```python
from build123d import *

# Parameters (mm, degrees)
BOSS_EXTRUDE1_DEPTH = 3
CUT_EXTRUDE1_REACH  = 27.671
SKETCH4_R           = 2.5


with BuildPart() as part:
    # Sketch2 → Boss-Extrude1 (new body)
    with BuildSketch(Plane.XY):
        with BuildLine():
            Line((-20, 5), (20, 5))
            ThreePointArc((20, 5), (25, 0), (20, -5))
            Line((20, -5), (-20, -5))
            ThreePointArc((-20, -5), (-25, 0), (-20, 5))
        make_face()
    extrude(amount=BOSS_EXTRUDE1_DEPTH)

    # Sketch4 → Cut-Extrude1 (cut, up to next)
    with BuildSketch(Plane.XY.offset(3), mode=Mode.PRIVATE) as cut_extrude1_sk1:
        with Locations((-20, 0)):
            Circle(SKETCH4_R)
    cut_extrude1_tool1 = extrude(cut_extrude1_sk1.sketch, amount=-CUT_EXTRUDE1_REACH, mode=Mode.PRIVATE) & part.part
    # Sketch4 → Cut-Extrude1 (cut, up to next)
    with BuildSketch(Plane.XY.offset(3), mode=Mode.PRIVATE) as cut_extrude1_sk2:
        with BuildLine():
            Line((11, 2.5), (18, 2.5))
            ThreePointArc((18, 2.5), (20.5, 0), (18, -2.5))
            Line((18, -2.5), (11, -2.5))
            ThreePointArc((11, -2.5), (8.5, 0), (11, 2.5))
        make_face()
    cut_extrude1_tool2 = extrude(cut_extrude1_sk2.sketch, amount=-CUT_EXTRUDE1_REACH, mode=Mode.PRIVATE) & part.part
    add(cut_extrude1_tool1.solids().sort_by_distance((-20, 0, 3))[0], mode=Mode.SUBTRACT)
    add(cut_extrude1_tool2.solids().sort_by_distance((14.5, 0, 3))[0], mode=Mode.SUBTRACT)


solid = part.part
```
Source: CAD feature listing. Evaluate the final solid. Frame: model axes, mm. A direction names the side the tool comes from. Round coordinates to 2 decimals unless told otherwise and drop trailing zeros. Loops run counter-clockwise (first coordinate to the right, second up) from the corner with the lowest first, then second, coordinate; pieces in that order, holes last.
1. Contact query for a flat-ended pin moving along its axis: pin 1 (6 mm diameter, centred on x = 9, y = -1, fed in from +Z). Output: stop coordinate, or through.
2. Section query B-B on y = 0. Output: boundary loops of the cut face in (x, z), and give its area (3 significant figures).
3. Section query A-A on z = 1.2. Output: boundary loops of the cut face in (x, y), and give its area (3 significant figures).
4. Access query for faces 4 (the flat face through (0, 5, 1)), 5 (the flat face through (15, -2.5, 2)). Directions: +Z, -Z, +X, -X, +Y, -Y. A direction counts if a zero-diameter tool reaches every point of the face in a straight line with its end or side. Return the directions, or none.
5. Section query C-C on x = -19.5. Output: boundary loops of the cut face in (y, z).
6. Section query D-D on y = -4. Output: boundary loops of the cut face in (x, z), and give its area (3 significant figures).
7. Ray query, L1, parallel to Y at x = 17.5, z = 1.4; L2, parallel to X at y = -1.5, z = 2.05; L3, parallel to Y at x = -21, z = 0.25. Return the intervals inside material, ascending.
8. Mould query, pull axis X, two halves, no side actions, for faces 1 (the cylindrical face through (25, 0, 1)), 2 (the flat face through (14, 2.5, 2)), 3 (the flat face through (0, -5, 1)). Classes: released by +X, released by -X, zero draft, split by the parting line, or undercut.
Answers below:
1. pin 1: stops at z = 3
2. outline: (-25, 0) - (-22.5, 0) - (-22.5, 3) - (-25, 3) - close; (-17.5, 0) - (8.5, 0) - (8.5, 3) - (-17.5, 3) - close; (20.5, 0) - (25, 0) - (25, 3) - (20.5, 3) - close
2. area: 99.0 mm2
3. outline: (-20, -5) - (20, -5) arc R5 ccw to (20, 5) - (-20, 5) arc R5 ccw to start; hole circle Ø5 at (-20, 0); hole (11, -2.5) - (18, -2.5) arc R2.5 ccw to (18, 2.5) - (11, 2.5) arc R2.5 ccw to start
3. area: 404 mm2
4. face 4: +Z, -Z, +X, -X, +Y
4. face 5: +Z, -Z
5. outline: (-5, 0) - (-2.45, 0) - (-2.45, 3) - (-5, 3) - close; (2.45, 0) - (5, 0) - (5, 3) - (2.45, 3) - close
6. outline: (-23, 0) - (23, 0) - (23, 3) - (-23, 3) - close
6. area: 138 mm2
7. L1: y = -5 to -2.5, 2.5 to 5
7. L2: x = -24.77 to -22, -18 to 9, 20 to 24.77
7. L3: y = -4.9 to -2.29, 2.29 to 4.9
8. face 1: released by +X
8. face 2: undercut
8. face 3: zero draft
